from build123d import *

# Parameters (mm, degrees)
SKETCH1_R           = 57.5
SKETCH1_R_2         = 39
SKETCH1_R_3         = 2
SKETCH1_R_4         = 2.5
BOSS_EXTRUDE1_DEPTH = 10
SKETCH2_R           = 2.5
CUT_EXTRUDE1_DEPTH  = 10
SKETCH4_R           = 5
SKETCH4_R_2         = 2.5
BOSS_EXTRUDE3_DEPTH = 0.4


with BuildPart() as part:
    # Sketch1 → Boss-Extrude1 (new body)
    with BuildSketch(Plane(origin=(0, 0, 0), x_dir=(1, 0, 0), z_dir=(0, 1, 0))):
        with Locations(Location((0, 0, 0), (0, 0, 270))):
            Circle(SKETCH1_R)
        with Locations(Location((0, 0, 0), (0, 0, 270))):
            Circle(SKETCH1_R_2, mode=Mode.SUBTRACT)
        with Locations(Location((0, 54, 0), (0, 0, 270))):
            Circle(SKETCH1_R_3, mode=Mode.SUBTRACT)
        with Locations(Location((27, 46.765371804, 0), (0, 0, 270))):
            Circle(SKETCH1_R_3, mode=Mode.SUBTRACT)
        with Locations(Location((46.765371804, 27, 0), (0, 0, 270))):
            Circle(SKETCH1_R_3, mode=Mode.SUBTRACT)
        with Locations(Location((54, 0, 0), (0, 0, 270))):
            Circle(SKETCH1_R_3, mode=Mode.SUBTRACT)
        with Locations(Location((46.765371804, -27, 0), (0, 0, 270))):
            Circle(SKETCH1_R_3, mode=Mode.SUBTRACT)
        with Locations(Location((27, -46.765371804, 0), (0, 0, 270))):
            Circle(SKETCH1_R_3, mode=Mode.SUBTRACT)
        with Locations(Location((0, -54, 0), (0, 0, 270))):
            Circle(SKETCH1_R_3, mode=Mode.SUBTRACT)
        with Locations(Location((-27, -46.765371804, 0), (0, 0, 270))):
            Circle(SKETCH1_R_3, mode=Mode.SUBTRACT)
        with Locations(Location((-46.765371804, -27, 0), (0, 0, 270))):
            Circle(SKETCH1_R_3, mode=Mode.SUBTRACT)
        with Locations(Location((-54, 0, 0), (0, 0, 270))):
            Circle(SKETCH1_R_3, mode=Mode.SUBTRACT)
        with Locations(Location((-46.765371804, 27, 0), (0, 0, 270))):
            Circle(SKETCH1_R_3, mode=Mode.SUBTRACT)
        with Locations(Location((-27, 46.765371804, 0), (0, 0, 270))):
            Circle(SKETCH1_R_3, mode=Mode.SUBTRACT)
        with Locations(Location((13.587999868, 50.71110588, 0), (0, 0, 270))):
            Circle(SKETCH1_R_4, mode=Mode.SUBTRACT)
        with Locations(Location((37.123106012, 37.123106012, 0), (0, 0, 270))):
            Circle(SKETCH1_R_4, mode=Mode.SUBTRACT)
        with Locations(Location((50.71110588, 13.587999868, 0), (0, 0, 270))):
            Circle(SKETCH1_R_4, mode=Mode.SUBTRACT)
        with Locations(Location((50.71110588, -13.587999868, 0), (0, 0, 270))):
            Circle(SKETCH1_R_4, mode=Mode.SUBTRACT)
        with Locations(Location((37.123106012, -37.123106012, 0), (0, 0, 270))):
            Circle(SKETCH1_R_4, mode=Mode.SUBTRACT)
        with Locations(Location((13.587999868, -50.71110588, 0), (0, 0, 270))):
            Circle(SKETCH1_R_4, mode=Mode.SUBTRACT)
        with Locations(Location((-13.587999868, -50.71110588, 0), (0, 0, 270))):
            Circle(SKETCH1_R_4, mode=Mode.SUBTRACT)
        with Locations(Location((-37.123106012, -37.123106012, 0), (0, 0, 270))):
            Circle(SKETCH1_R_4, mode=Mode.SUBTRACT)
        with Locations(Location((-50.71110588, -13.587999868, 0), (0, 0, 270))):
            Circle(SKETCH1_R_4, mode=Mode.SUBTRACT)
        with Locations(Location((-50.71110588, 13.587999868, 0), (0, 0, 270))):
            Circle(SKETCH1_R_4, mode=Mode.SUBTRACT)
        with Locations(Location((-37.123106012, 37.123106012, 0), (0, 0, 270))):
            Circle(SKETCH1_R_4, mode=Mode.SUBTRACT)
        with Locations(Location((-13.587999868, 50.71110588, 0), (0, 0, 270))):
            Circle(SKETCH1_R_4, mode=Mode.SUBTRACT)
    extrude(amount=BOSS_EXTRUDE1_DEPTH)

    # Sketch2 → Cut-Extrude1 (cut)
    with BuildSketch(Plane(origin=(0, 10, 0), x_dir=(1, 0, 0), z_dir=(0, 1, 0))):
        with Locations(Location((0, 45, 0), (0, 0, 270))):
            Circle(SKETCH2_R)
        with Locations(Location((17.220754456, 41.574578963, 0), (0, 0, 270))):
            Circle(SKETCH2_R)
        with Locations(Location((31.819805153, 31.819805153, 0), (0, 0, 270))):
            Circle(SKETCH2_R)
        with Locations(Location((41.574578963, 17.220754456, 0), (0, 0, 270))):
            Circle(SKETCH2_R)
        with Locations(Location((45, 0, 0), (0, 0, 270))):
            Circle(SKETCH2_R)
        with Locations(Location((41.574578963, -17.220754456, 0), (0, 0, 270))):
            Circle(SKETCH2_R)
        with Locations(Location((31.819805153, -31.819805153, 0), (0, 0, 270))):
            Circle(SKETCH2_R)
        with Locations(Location((17.220754456, -41.574578963, 0), (0, 0, 270))):
            Circle(SKETCH2_R)
        with Locations(Location((0, -45, 0), (0, 0, 270))):
            Circle(SKETCH2_R)
        with Locations(Location((-17.220754456, -41.574578963, 0), (0, 0, 270))):
            Circle(SKETCH2_R)
        with Locations(Location((-31.819805153, -31.819805153, 0), (0, 0, 270))):
            Circle(SKETCH2_R)
        with Locations(Location((-41.574578963, -17.220754456, 0), (0, 0, 270))):
            Circle(SKETCH2_R)
        with Locations(Location((-45, 0, 0), (0, 0, 270))):
            Circle(SKETCH2_R)
        with Locations(Location((-41.574578963, 17.220754456, 0), (0, 0, 270))):
            Circle(SKETCH2_R)
        with Locations(Location((-31.819805153, 31.819805153, 0), (0, 0, 270))):
            Circle(SKETCH2_R)
        with Locations(Location((-17.220754456, 41.574578963, 0), (0, 0, 270))):
            Circle(SKETCH2_R)
    extrude(amount=-CUT_EXTRUDE1_DEPTH, mode=Mode.SUBTRACT)

    # Sketch4 → Boss-Extrude3 (add)
    # profile 1 of 16: a face of its own
    with BuildSketch(Plane(origin=(0, 0, 0), x_dir=(1, 0, 0), z_dir=(0, 1, 0))):
        with Locations(Location((0, 45, 0), (0, 0, 270))):
            Circle(SKETCH4_R)
        with Locations(Location((0, 45, 0), (0, 0, 270))):
            Circle(SKETCH4_R_2, mode=Mode.SUBTRACT)
    # profile 2 of 16: a face of its own
    with BuildSketch(Plane(origin=(0, 0, 0), x_dir=(1, 0, 0), z_dir=(0, 1, 0))):
        with Locations(Location((17.220754456, 41.574578963, 0), (0, 0, 270))):
            Circle(SKETCH4_R)
        with Locations(Location((17.220754456, 41.574578963, 0), (0, 0, 270))):
            Circle(SKETCH4_R_2, mode=Mode.SUBTRACT)
    # profile 3 of 16: a face of its own
    with BuildSketch(Plane(origin=(0, 0, 0), x_dir=(1, 0, 0), z_dir=(0, 1, 0))):
        with Locations(Location((31.819805153, 31.819805153, 0), (0, 0, 270))):
            Circle(SKETCH4_R)
        with Locations(Location((31.819805153, 31.819805153, 0), (0, 0, 270))):
            Circle(SKETCH4_R_2, mode=Mode.SUBTRACT)
    # profile 4 of 16: a face of its own
    with BuildSketch(Plane(origin=(0, 0, 0), x_dir=(1, 0, 0), z_dir=(0, 1, 0))):
        with Locations(Location((41.574578963, 17.220754456, 0), (0, 0, 270))):
            Circle(SKETCH4_R)
        with Locations(Location((41.574578963, 17.220754456, 0), (0, 0, 270))):
            Circle(SKETCH4_R_2, mode=Mode.SUBTRACT)
    # profile 5 of 16: a face of its own
    with BuildSketch(Plane(origin=(0, 0, 0), x_dir=(1, 0, 0), z_dir=(0, 1, 0))):
        with Locations(Location((45, 0, 0), (0, 0, 270))):
            Circle(SKETCH4_R)
        with Locations(Location((45, 0, 0), (0, 0, 270))):
            Circle(SKETCH4_R_2, mode=Mode.SUBTRACT)
    # profile 6 of 16: a face of its own
    with BuildSketch(Plane(origin=(0, 0, 0), x_dir=(1, 0, 0), z_dir=(0, 1, 0))):
        with Locations(Location((41.574578963, -17.220754456, 0), (0, 0, 270))):
            Circle(SKETCH4_R)
        with Locations(Location((41.574578963, -17.220754456, 0), (0, 0, 270))):
            Circle(SKETCH4_R_2, mode=Mode.SUBTRACT)
    # profile 7 of 16: a face of its own
    with BuildSketch(Plane(origin=(0, 0, 0), x_dir=(1, 0, 0), z_dir=(0, 1, 0))):
        with Locations(Location((31.819805153, -31.819805153, 0), (0, 0, 270))):
            Circle(SKETCH4_R)
        with Locations(Location((31.819805153, -31.819805153, 0), (0, 0, 270))):
            Circle(SKETCH4_R_2, mode=Mode.SUBTRACT)
    # profile 8 of 16: a face of its own
    with BuildSketch(Plane(origin=(0, 0, 0), x_dir=(1, 0, 0), z_dir=(0, 1, 0))):
        with Locations(Location((17.220754456, -41.574578963, 0), (0, 0, 270))):
            Circle(SKETCH4_R)
        with Locations(Location((17.220754456, -41.574578963, 0), (0, 0, 270))):
            Circle(SKETCH4_R_2, mode=Mode.SUBTRACT)
    # profile 9 of 16: a face of its own
    with BuildSketch(Plane(origin=(0, 0, 0), x_dir=(1, 0, 0), z_dir=(0, 1, 0))):
        with Locations(Location((0, -45, 0), (0, 0, 270))):
            Circle(SKETCH4_R)
        with Locations(Location((0, -45, 0), (0, 0, 270))):
            Circle(SKETCH4_R_2, mode=Mode.SUBTRACT)
    # profile 10 of 16: a face of its own
    with BuildSketch(Plane(origin=(0, 0, 0), x_dir=(1, 0, 0), z_dir=(0, 1, 0))):
        with Locations(Location((-17.220754456, -41.574578963, 0), (0, 0, 270))):
            Circle(SKETCH4_R)
        with Locations(Location((-17.220754456, -41.574578963, 0), (0, 0, 270))):
            Circle(SKETCH4_R_2, mode=Mode.SUBTRACT)
    # profile 11 of 16: a face of its own
    with BuildSketch(Plane(origin=(0, 0, 0), x_dir=(1, 0, 0), z_dir=(0, 1, 0))):
        with Locations(Location((-31.819805153, -31.819805153, 0), (0, 0, 270))):
            Circle(SKETCH4_R)
        with Locations(Location((-31.819805153, -31.819805153, 0), (0, 0, 270))):
            Circle(SKETCH4_R_2, mode=Mode.SUBTRACT)
    # profile 12 of 16: a face of its own
    with BuildSketch(Plane(origin=(0, 0, 0), x_dir=(1, 0, 0), z_dir=(0, 1, 0))):
        with Locations(Location((-41.574578963, -17.220754456, 0), (0, 0, 270))):
            Circle(SKETCH4_R)
        with Locations(Location((-41.574578963, -17.220754456, 0), (0, 0, 270))):
            Circle(SKETCH4_R_2, mode=Mode.SUBTRACT)
    # profile 13 of 16: a face of its own
    with BuildSketch(Plane(origin=(0, 0, 0), x_dir=(1, 0, 0), z_dir=(0, 1, 0))):
        with Locations(Location((-45, 0, 0), (0, 0, 270))):
            Circle(SKETCH4_R)
        with Locations(Location((-45, 0, 0), (0, 0, 270))):
            Circle(SKETCH4_R_2, mode=Mode.SUBTRACT)
    # profile 14 of 16: a face of its own
    with BuildSketch(Plane(origin=(0, 0, 0), x_dir=(1, 0, 0), z_dir=(0, 1, 0))):
        with Locations(Location((-41.574578963, 17.220754456, 0), (0, 0, 270))):
            Circle(SKETCH4_R)
        with Locations(Location((-41.574578963, 17.220754456, 0), (0, 0, 270))):
            Circle(SKETCH4_R_2, mode=Mode.SUBTRACT)
    # profile 15 of 16: a face of its own
    with BuildSketch(Plane(origin=(0, 0, 0), x_dir=(1, 0, 0), z_dir=(0, 1, 0))):
        with Locations(Location((-31.819805153, 31.819805153, 0), (0, 0, 270))):
            Circle(SKETCH4_R)
        with Locations(Location((-31.819805153, 31.819805153, 0), (0, 0, 270))):
            Circle(SKETCH4_R_2, mode=Mode.SUBTRACT)
    # profile 16 of 16: a face of its own
    with BuildSketch(Plane(origin=(0, 0, 0), x_dir=(1, 0, 0), z_dir=(0, 1, 0))):
        with Locations(Location((-17.220754456, 41.574578963, 0), (0, 0, 270))):
            Circle(SKETCH4_R)
        with Locations(Location((-17.220754456, 41.574578963, 0), (0, 0, 270))):
            Circle(SKETCH4_R_2, mode=Mode.SUBTRACT)
    extrude(amount=-BOSS_EXTRUDE3_DEPTH)


solid = part.part
Input: part model. Units: mm. Frame: model coordinates. A direction names the side the tool comes from. Round coordinates to 2 decimals unless told otherwise and drop trailing zeros.
1) Draft query along X for faces 3 (the cylindrical face through (-56.133, 4.93, -12.465)), 4 (the cylindrical face through (-53.15, 4.93, -14.13)), 5 (the flat face through (-18, -0.4, 39)). Return one class per face: pulls with the +X half, pulls with the -X half, needs draft (parallel to the pull), parting line crosses it, or undercut.
2) Reachability of faces 1 (the cylindrical face through (43.076, -0.197, -12.452)), 2 (the flat face through (-47, -0.4, 2)) from +Z, -Z, +X, -X, +Y, -Y: full face, straight path, thin tool, end or side. Return the list, or none.
3) Ray query, L1, parallel to X at y = 5.75, z = 0; L2, parallel to X at y = 3, z = -18.5; L3, parallel to X at y = 3.25, z = -28. Return the intervals inside material, ascending.
4) Contact query for flat-ended pins moving along their axis: P1, Ø4, axis at x = -38, y = 5, coming from the -Z side; P2, Ø2, axis at x = -42, y = 1.5, coming from the +Z side; P3, Ø8, axis at x = 50.71, z = -13.59, coming from the -Y side. Output: stop coordinate, or through.
5) Cut plane A-A (z = 0). Count the separate pieces of the cut face and the enclosed holes in it, then the cut area to 3 significant figures.
Geometry says:
1. face 3: parting line crosses it
1. face 4: undercut
1. face 5: needs draft
2. face 1: -Y
2. face 2: +Z, -Z, +X, -X, -Y
3. L1: x = -57.5 to -56, -52 to -47.5, -42.5 to -39, 39 to 42.5, 47.5 to 52, 56 to 57.5
3. L2: x = -54.44 to -43.72, -39.43 to -34.33, 34.33 to 39.43, 43.72 to 54.44
3. L3: x = -50.22 to -48.5, -45.03 to -27.15, 27.15 to 45.03, 48.5 to 50.22
4. P1: stops at z = -44.84
4. P2: stops at z = 40.31
4. P3: stops at y = 0
5. separate pieces: 6
5. enclosed holes: 0
5. area: 194 mm2
